Can you work these out from the model? Positions are in its coordinate system, mm. Face numbers are marked on the shaded views. A direction names the side the tool comes from. Give positions to 0.01 mm unless a question says otherwise; leave off trailing zeros. Order: outer loops, then holes, each group sorted by start corner. A loop starts at its lowest first (then second) coordinate and runs counter-clockwise, first axis right, second up. Notation, with made-up numbers: (53.25, 77) - (104.25, 77) arc R38 cw to (104.25, 116) - close; hole circle Ø11 at (65, -7). An arc over 180 degrees is marked (long way). Return JSON: item names as keys, results as strings.
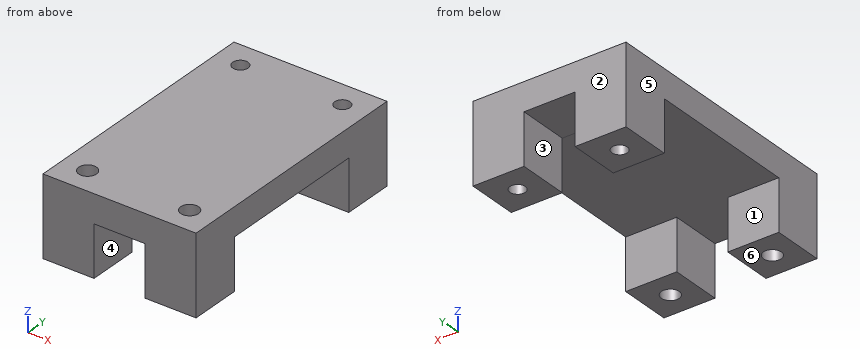
```python
from build123d import *

# Parameters (mm, degrees)
F1_DEPTH  = 10
F2_R      = 1.5
F3_DEPTH  = 16
F5_W      = 30
F5_H      = 29.9720647931
F5_H_2    = 10
F5_R      = 1.5
F6_DEPTH  = 5.53592
F7_W      = 10
F7_H      = 10
F8_DEPTH  = 10
F9_R      = 1.75
F10_DEPTH = 25


with BuildPart() as f1:
    # F0 (on Front) → F1 (new body)
    with BuildSketch(Plane.XZ):
        Polygon((-5, 5), (5, 5), (5, -5), (15, -5), (15, 5), (15, 7.7369394712), (15, 10.5359181762), (10.6142175943, 10.5359181762), (0, 10.5359181762), (-10.6142175943, 10.5359181762), (-15, 10.5359181762), (-15, 7.7369394712), (-15, 5), (-15, -5), (-5, -5), align=None)
    extrude(amount=F1_DEPTH)

    # F2 (on face) → F3 (cut)
    with BuildSketch(Plane(origin=(0, 0, -5), x_dir=(1, 0, 0), z_dir=(0, 0, -1))):
        with Locations((10, 5)):
            Circle(F2_R)
        with Locations((-10, 5)):
            Circle(F2_R)
    extrude(amount=-F3_DEPTH, mode=Mode.SUBTRACT)

    # F5 (on face) → F6 (join)
    with BuildSketch(Plane.XY.offset(10.5359181762)):
        with Locations((0, -24.9860323966)):
            Rectangle(F5_W, F5_H)
        with Locations((0, -44.9720647931)):
            Rectangle(F5_W, F5_H_2)
        with Locations((-10, -44.9720647931)):
            Circle(F5_R, mode=Mode.SUBTRACT)
        with Locations((10, -44.9720647931)):
            Circle(F5_R, mode=Mode.SUBTRACT)
    extrude(amount=-F6_DEPTH)

    # F7 (on face) → F8 (join)
    with BuildSketch(Plane(origin=(0, 0, 5), x_dir=(1, 0, 0), z_dir=(0, 0, -1))):
        with Locations((10, 44.9720647931)):
            Rectangle(F7_W, F7_H)
        with Locations((-10, 44.9720647931)):
            Rectangle(F7_W, F7_H)
    extrude(amount=F8_DEPTH)

    # F9 (on face) → F10 (cut)
    with BuildSketch(Plane(origin=(0, 0, -5), x_dir=(1, 0, 0), z_dir=(0, 0, -1))):
        with Locations((-10, 44.9720647931)):
            Circle(F9_R)
        with Locations((10, 44.9720647931)):
            Circle(F9_R)
    extrude(amount=-F10_DEPTH, mode=Mode.SUBTRACT)


solid = f1.part
```
1. Suppose I cut it at A-A (y = -5). List the corners of the cut face in (x, z) for me, plus the area to 3 significant figures.
Checks:
{"outline": "(-15, -5) - (-11.5, -5) - (-11.5, 10.54) - (-15, 10.54) - close; (-8.5, -5) - (-5, -5) - (-5, 5) - (5, 5) - (5, -5) - (8.5, -5) - (8.5, 10.54) - (-8.5, 10.54) - close; (11.5, -5) - (15, -5) - (15, 10.54) - (11.5, 10.54) - close", "area": "273 mm^2"}
2. For pin 1 Ø2.5 at (x, y) = (-10, -5) entering from -Z; pin 2 Ø11 at (x, y) = (2.5, -4.5) entering from -Z; pin 3 Ø2 at (x, y) = (0.5, -17.5) entering from -Z, each with a flat end and sliding along its axis, tell me the tip position at first contact or that it passes through.
Checks:
{"pin 1": "through", "pin 2": "z = -5", "pin 3": "z = 5"}
3. Suppose I cut it at B-B (x = 10). List the corners of the cut face in (y, z) for me, plus the area to 3 significant figures.
Checks:
{"outline": "(-49.97, -5) - (-46.72, -5) - (-46.72, 10.54) - (-49.97, 10.54) - close; (-43.22, -5) - (-39.97, -5) - (-39.97, 5) - (-10, 5) - (-10, -5) - (-6.5, -5) - (-6.5, 10.54) - (-43.22, 10.54) - close; (-3.5, -5) - (0, -5) - (0, 10.54) - (-3.5, 10.54) - close", "area": "376 mm^2"}
4. Suppose I cut it at C-C (z = 2.75). List the corners of the cut face in (x, y) for me, plus the area to 3 significant figures.
Checks:
{"outline": "(-15, -49.97) - (-5, -49.97) - (-5, -39.97) - (-15, -39.97) - close; (-15, -10) - (-5, -10) - (-5, 0) - (-15, 0) - close; (5, -49.97) - (15, -49.97) - (15, -39.97) - (5, -39.97) - close; (5, -10) - (15, -10) - (15, 0) - (5, 0) - close; hole circle Ø3.5 at (-10, -44.97); hole circle Ø3 at (-10, -5); hole circle Ø3.5 at (10, -44.97); hole circle Ø3 at (10, -5)", "area": "367 mm^2"}
5. If I drill on L1, parallel to Y at x = 10, z = 2.25; L2, parallel to X at y = -5, z = -0.75; L3, parallel to X at y = -40.5, z = 0.25, over which ranges is the centre line in solid material (lowest first)? Write a range as [from, to].
Checks:
{"L1": "[-49.97, -46.72], [-43.22, -39.97], [-10, -6.5], [-3.5, 0]", "L2": "[-15, -11.5], [-8.5, -5], [5, 8.5], [11.5, 15]", "L3": "[-15, -5], [5, 15]"}
6. On a 3-axis mill with a long thin cutter (end or side, diameter ignored), from which of +Z, -Z, +X, -X, +Y, -Y can I reach the whole of each face in a straight line? I mean the marked faces 1, 2 and 3. Say none if no direction works.
Checks:
{"face 1": "-Z, +X, -X", "face 2": "+Z, -Z, +X, -X, +Y", "face 3": "-Z, +Y, -Y"}
7. Thinking about a two-plate mould opening in X: for the marked faces 4, 5 and 6, which applies, +X half, -X half, draft (parallel to the pull), parting line (faces both ways), or undercut?
Checks:
{"face 4": "undercut", "face 5": "-X half", "face 6": "draft"}
